Autodesk Fusion 360 part; units mm, degrees
sketch "Sketch1" plane through (0, 0, 0) normal (0, 0, 1) x (1, 0, 0)
  circle A0 centre (-50, 0) radius 9.5
  arc A1 (-29.5, -18) -> (-31, -19.5) centre (-29.5, -19.5) ccw
  arc A2 (-31, 19.5) -> (-29.5, 18) centre (-29.5, 19.5) ccw
  line L0 (-31, 43) -> (-31, 19.5)
  line L1 (-31, -19.5) -> (-31, -43)
  line L2 (-24, 5) -> (-24, -5)
  line L3 (-50, 43) -> (-50, 44)
  line L4 (-44, 44) -> (2.7447, 44)
  line L5 (42, 44) -> (42, 43)
  line L6 (-50, -43) -> (-50, -44)
  line L7 (-31, -43) -> (-31, -44)
  line L8 (-24, -43) -> (-24, -44)
  line L9 (-13, -43) -> (-13, -44)
  line L10 (42, -43) -> (42, -44)
  line L11 (-13, 43) -> (-13, 44)
  line L12 (-24, 43) -> (-24, 44)
  line L13 (-31, 43) -> (-31, 44)
  line L14 (-31, 44) -> (-44, 44)
  arc A3 (-47.4091, 18.8225) -> (-47.4091, -18.8225) centre (-50, 0) ccw
  line L15 (-44, 44) -> (-44, 21.7945)
  line L16 (-44, -21.7945) -> (-44, -44)
  arc A4 (-47.4091, 18.8225) -> (-44, 21.7945) centre (-47, 21.7945) ccw
  arc A5 (-44, -21.7945) -> (-47.4091, -18.8225) centre (-47, -21.7945) ccw
  line L17 (-31, 44) -> (0, 44)
  line L18 (0, 44) -> (0, 43.393)
  circle A6 centre (0, 27) radius 5
  circle A7 centre (0, -27) radius 5
  line L19 (0, 44) -> (2.7426, 44)
  line L20 (36, 0) -> (36, 5)
  line L21 (36, 5) -> (-29.5, 5)
  line L22 (36, 5) -> (36, -5)
  line L23 (36, -5) -> (-29.5, -5)
  line L24 (45.5, -44) -> (42, -44)
  line L25 (42.7175, -6.7175) -> (7.3388, -42.0962)
  arc A8 (2.7426, -44) -> (7.3388, -42.0962) centre (2.7426, -37.5) ccw
  arc A9 (0, -31.607) -> (-0.6526, -31.9572) centre (2.7426, -37.5) ccw
  line L26 (0, -44) -> (0, -43.393)
  line L27 (0, -32) -> (0, -31.607)
  line L28 (-44, -44) -> (2.7426, -44)
  line L29 (42.7175, 6.7175) -> (7.3388, 42.0962)
  arc A10 (7.3388, 42.0962) -> (2.7406, 44) centre (2.7426, 37.5) ccw
  arc A11 (42.7175, -6.7175) -> (42.7175, 6.7175) centre (36, 0) ccw
  line L30 (36, 5) -> (36, -5)
  line L31 (36, -9.5) -> (36, -13.435)
  line L32 (-29.5, 18) -> (-29.5, 5)
  line L33 (-29.5, -5) -> (-29.5, -18)
  dimension "d10" = 19
  dimension "d11" = 19
  dimension "d18" = 3
  dimension "d19" = 3
  dimension "d22" = 92
  dimension "d25" = 88
  dimension "d26" = 13
  dimension "d28" = 6
  dimension "d29" = 6
  dimension "d30" = 20
  dimension "d31" = 31
  dimension "d32" = 17
  dimension "d33" = 17
  dimension "d34" = 10
  dimension "d35" = 10
  dimension "d38" = 19
  dimension "d43" = 13
  dimension "d47" = 13
extrude "Extrude5" add sketch "Sketch1" along normal blind 40 contours A1 A2 L0 L1 L2 L4 L7 L13 L14 A3 L15 L16 A4 A5 L21 L23 L28 L32 L33
extrude "Extrude6" add sketch "Sketch1" along normal blind 10 contours A1 A2 L0 L1 L4 L7 L13 L17 L19 L20 L21 L22 L23 L25 A8 L28 L29 A10 A11 L30 L32 L33
extrude "Extrude7" add sketch "Sketch1" along normal blind 40 contours L2 L20 L21 L22 L23 L30
sketch "Sketch3" plane through (0, -5, 0) normal (0, -1, 0) x (1, 0, 0)
  line L0 (-29.5, 10) -> (36, 10)
  line L1 (36, 10) -> (36, 40)
  line L2 (36, 40) -> (-29.5, 40)
  line L3 (-29.5, 40) -> (-29.5, 10)
  line L4 (-29.5, 40) -> (-25.5, 40)
  line L5 (-25.5, 40) -> (36, 10)
  dimension "d62" = 4
extrude "Extrude8" cut sketch "Sketch3" against normal blind 10 contours L1 L2 L5
extrude "Extrude2" [suppressed]
extrude "Extrude1" [suppressed]
extrude "Extrude3" [suppressed]
sketch "Sketch2" plane through (0, -5, 0) normal (0, -1, 0) x (1, 0, 0)
  line L0 (-29.5, 10) -> (36, 10)
  line L1 (36, 10) -> (36, 40)
  line L2 (36, 40) -> (-29.5, 40)
  line L3 (-29.5, 40) -> (-29.5, 10)
  line L4 (-29.5, 40) -> (36, 10)
extrude "Extrude4" [suppressed]
Verification items for the finished model (mm, model axes). A direction names the side the tool comes from. Give positions to 0.01 mm unless a question says otherwise; leave off trailing zeros. Order: outer loops, then holes, each group sorted by start corner. A loop starts at its lowest first (then second) coordinate and runs counter-clockwise, first axis right, second up. Notation, with made-up numbers: M 22.25,-8 L 36.25,-8 A13 ccw 36.25,-4 Z; hole C -10.75,87.25 d6. An arc over 180 degrees is marked long. Answer in a Markdown table with one row per item. Add a question column.
Item 1: Scan lines: probe 1 along Y at (x, z) = (0, 8); probe 2 along Y at (x, z) = (-50, 23); probe 3 along X at (y, z) = (39.5, 34.5). Record each from-to range of solid material in increasing order. Write a range as from..to.
Item 2: Section check A-A, the plane x = -50. Enter the section's corners in (y, z), and give its area (3 significant figures).
Item 3: Section check B-B, the plane z = 19.5. Enter the section's corners in (x, y) (1 decimal), and give its area (3 significant figures).
Item 4: Section check D-D, the plane x = 21. Enter the section's corners in (y, z) (3 decimals), and give its area (3 significant figures).
Item 5: Mould release check, pull along Y, two halves, no side actions. Record for faces 6 (the flat face through (-31.3, 44, 15.3)), 7 (the flat face through (-44, -33, 20)), 8 (the cylindrical face through (-1.08, -22.12, 4.93)): released by +Y, released by -Y, zero draft, split by the parting line, or undercut.
Item 6: Section check C-C, the plane y = 25. Enter the section's corners in (x, z) (3 decimals).
Item 7: Gauge pin test, flat ends, axial feed: pin 1 (1 mm diameter, centred on y = -6.5, z = 24, fed in from -X); pin 2 (4 mm diameter, centred on x = 19, y = 32.5, fed in from +Z); pin 3 (9 mm diameter, centred on x = -10, z = 27, fed in from +Y). Record the tip position at first contact, or that the pin passes through.
Item 8: Tool access check on faces 1 (the flat face through (-29.5, 12, 25)), 2 (the flat face through (-29.5, -11, 25)), 3 (the flat face through (-38, 1, 40)), 4 (the flat face through (-13, 1, 0)), 5 (the flat face through (-44, 33, 20)). Record the directions out of +Z, -Z, +X, -X, +Y, -Y that give a thin tool (end or side, any length) a straight path to the whole face; none if there is none.
Filled sheet:
| question | item | result |
|---|---|---|
| 1 | probe 1 | y = -44..-32, -22..22, 32..44 |
| 1 | probe 2 | y = -19..-9.5, 9.5..19 |
| 1 | probe 3 | x = -44..-31 |
| 2 | outline | M -19,0 L -9.5,0 L -9.5,40 L -19,40 Z; M 9.5,0 L 19,0 L 19,40 L 9.5,40 Z |
| 2 | area | 760 mm^2 |
| 3 | outline | M -47.4,-18.8 A3 cw -44,-21.8 L -44,-44 L -31,-44 L -31,-19.5 A1.5 cw -29.5,-18 L -29.5,-5 L 16.5,-5 L 16.5,5 L -29.5,5 L -29.5,18 A1.5 cw -31,19.5 L -31,44 L -44,44 L -44,21.8 A3 cw -47.4,18.8 A19 ccw long Z; hole C -50,0 d19 |
| 3 | area | 2,170 mm^2 |
| 4 | outline | M -28.435,0 L 28.435,0 L 28.435,10 L 5,10 L 5,17.317 L -5,17.317 L -5,10 L -28.435,10 Z |
| 4 | area | 642 mm^2 |
| 5 | face 6 | released by +Y |
| 5 | face 7 | zero draft |
| 5 | face 8 | undercut |
| 6 | outline | M -44,0 L -4.583,0 L -4.583,10 L -31,10 L -31,40 L -44,40 Z; M 4.583,0 L 24.435,0 L 24.435,10 L 4.583,10 Z |
| 7 | pin 1 | stops at x = -68.03 |
| 7 | pin 2 | stops at z = 10 |
| 7 | pin 3 | stops at y = 5 |
| 8 | face 1 | +Z, +X, +Y |
| 8 | face 2 | +Z, +X, -Y |
| 8 | face 3 | +Z, +X, -X, +Y, -Y |
| 8 | face 4 | -Z, +X, -X, +Y, -Y |
| 8 | face 5 | +Z, -Z, -X, +Y |
